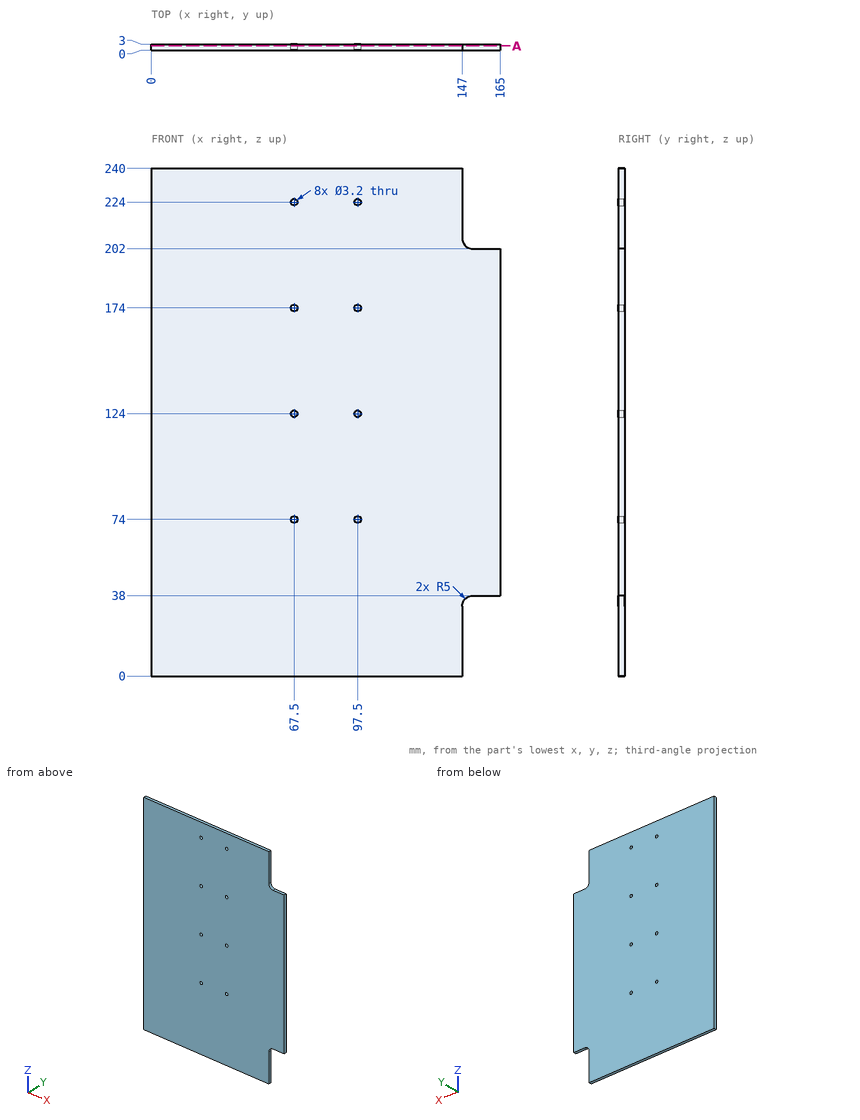
Source: three-view drawing plus pictorial views. Frame: mm from the lowest corner of the part. Round coordinates to 2 decimals unless told otherwise and drop trailing zeros. Write each question's results on one line, items separated by ' | '.
Q1. Section query A-A (y = 2.1). State how many separate pieces and enclosed holes the cut face has, and give its area (3 significant figures).
Results:
separate pieces: 1 | enclosed holes: 8 | area: 38,200 mm^2
Q2. Line query: line 1 along X through (y, z) = (1.1, 124); line 2 along Z through (x, y) = (97.5, 1.9); line 3 along X through (y, z) = (2.1, 224). Output: solid intervals per line, ascending.
Results:
line 1: x = 0 to 65.9, 69.1 to 95.9, 99.1 to 165 | line 2: z = 0 to 72.4, 75.6 to 122.4, 125.6 to 172.4, 175.6 to 222.4, 225.6 to 240 | line 3: x = 0 to 65.9, 69.1 to 95.9, 99.1 to 147
Q3. Pin query (flat end, axial travel): P1, Ø1.5, axis at x = 157.5, y = 1.5, coming from the -Z side; P2, Ø0.9, axis at y = 1.5, z = 218.5, coming from the +X side. Return the tip coordinate at first contact, or that it passes through.
Results:
P1: stops at z = 38 | P2: stops at x = 147
